Part model, mm, in its own coordinate system. A direction names the side the tool comes from. Round coordinates to 2 decimals unless told otherwise and drop trailing zeros. Loops run counter-clockwise (first coordinate to the right, second up) from the corner with the lowest first, then second, coordinate; pieces in that order, holes last. Notation, with made-up numbers: (-2, -32.5) - (30, -32.5) arc R7 cw to (30, -26.5) - close; hole circle Ø9 at (65.5, -38). An arc over 180 degrees is marked (long way). Put each result on its own line as item: value.
from build123d import *

# Parameters (mm, degrees)
EXTRUDE_1_DEPTH     = 65
MM_1_D              = 8
SKETCH_5_R          = 4.5
CUT_EXTRUDE_1_DEPTH = 89.741196746
SKETCH_6_R          = 7.5
CUT_EXTRUDE_2_DEPTH = 10
SKETCH_7_R          = 3.4
SKETCH_7_R_2        = 4
CUT_EXTRUDE_3_DEPTH = 24


with BuildPart() as part:
    # 草图1 → 凸台-拉伸1 (new body)
    with BuildSketch(Plane.XY):
        Polygon((-30, 44.5), (-30, 25), (0, 25), (0, 0), (-55, 0), (-55, 44.5), align=None)
    extrude(amount=EXTRUDE_1_DEPTH)

    # 大小mm 暗销孔1 (through all)
    with Locations(Plane(origin=(0, 25, 0), x_dir=(1, 0, 0), z_dir=(0, 1, 0))):
        with Locations((-12.5, -10), (-12.5, -40)):
            Hole(MM_1_D / 2)

    # 草图5 → 切除-拉伸1 (cut, through all)
    with BuildSketch(Plane(origin=(0, 25, 0), x_dir=(1, 0, 0), z_dir=(0, 1, 0))):
        with Locations(Location((-12.5, -25, 0), (0, 0, 270))):
            Circle(SKETCH_5_R)
        with Locations(Location((-12.5, -55, 0), (0, 0, 270))):
            Circle(SKETCH_5_R)
    extrude(amount=-CUT_EXTRUDE_1_DEPTH, mode=Mode.SUBTRACT)

    # 草图6 → 切除-拉伸2 (cut)
    with BuildSketch(Plane.XZ):
        with Locations((-12.5, 55)):
            Circle(SKETCH_6_R)
        with Locations((-12.5, 25)):
            Circle(SKETCH_6_R)
    extrude(amount=-CUT_EXTRUDE_2_DEPTH, mode=Mode.SUBTRACT)

    # 草图7 → 切除-拉伸3 (cut)
    with BuildSketch(Plane.ZY.offset(55)):
        with Locations((10, 32)):
            Circle(SKETCH_7_R)
        with Locations((25, 32)):
            Circle(SKETCH_7_R_2)
        with Locations((40, 32)):
            Circle(SKETCH_7_R)
        with Locations((55, 32)):
            Circle(SKETCH_7_R_2)
    extrude(amount=-CUT_EXTRUDE_3_DEPTH, mode=Mode.SUBTRACT)


solid = part.part
1. Band-saw the part on C-C (z = 25). List the corners of the cut face in (x, y).
A:
outline: (-55, 0) - (-20, 0) - (-20, 10) - (-17, 10) - (-17, 25) - (-30, 25) - (-30, 44.5) - (-55, 44.5) - (-55, 36) - (-31, 36) - (-31, 28) - (-55, 28) - close; (-8, 10) - (-5, 10) - (-5, 0) - (0, 0) - (0, 25) - (-8, 25) - close
2. Tool access for faces 4 (the flat face through (-33, 18, 0)), 5 (the flat face through (-43, 44.5, 32)), 6 (the flat face through (-7.6, 10, 25.1)), 7 (the cylindrical face through (-43.17, 30.7, 43.14)), 8 (the flat face through (-15, 25, 32)): list every direction of +Z, -Z, +X, -X, +Y, -Y with a clear straight run to the whole face (end or side of a thin tool).
A:
face 4: -Z, +X, -X, +Y, -Y
face 5: +Z, -Z, +X, -X, +Y
face 6: -Y
face 7: -X
face 8: +Z, -Z, +X, +Y
3. Pin check, flat tips, straight feed: P1, Ø12, axis at x = -12.5, z = 55, coming from the -Y side; P2, Ø4, axis at y = 33.5, z = 54, coming from the -X side; P3, Ø15.5, axis at y = 37.5, z = 47, coming from the +X side. Stop position of each tip, or through.
A:
P1: stops at y = 10
P2: stops at x = -31
P3: stops at x = -30
4. Two-plate mould, pull along X, no slides. Class faces 1 (the cylindrical face through (-13.476, 4.93, 32.436)), 2 (the flat face through (0, 13, 32)), 3 (the flat face through (-27, 0, 32)): pulls with the +X half, pulls with the -X half, needs draft (parallel to the pull), parting line crosses it, or undercut.
A:
face 1: undercut
face 2: pulls with the +X half
face 3: needs draft
5. Band-saw the part on D-D (x = -47.5). List the corners of the cut face in (y, z).
A:
outline: (0, 0) - (44.5, 0) - (44.5, 65) - (0, 65) - close; hole circle Ø8 at (32, 25); hole circle Ø8 at (32, 55); hole circle Ø6.8 at (32, 10); hole circle Ø6.8 at (32, 40)
6. Band-saw the part on B-B (y = 19). List the corners of the cut face in (x, z), plus the area to 3 significant figures.
A:
outline: (-55, 0) - (0, 0) - (0, 65) - (-55, 65) - close; hole circle Ø9 at (-12.5, 25); hole circle Ø9 at (-12.5, 55); hole circle Ø8 at (-12.5, 10); hole circle Ø8 at (-12.5, 40)
area: 3,350 mm²
7. Probe line 1 along X through (y, z) = (15, 40); line 2 along Y through (x, z) = (-39.5, 40); line 3 along Z through (x, y) = (-12, 8). List the from-to ranges inside material, lowest first. Write a range as [from, to].
A:
line 1: x = [-55, -16.5], [-8.5, 0]
line 2: y = [0, 28.6], [35.4, 44.5]
line 3: z = [0, 6.03], [13.97, 17.52], [32.48, 36.03], [43.97, 47.52], [62.48, 65]
8. Band-saw the part on A-A (x = -12.5). List the corners of the cut face in (y, z), plus the area to 3 significant figures.
A:
outline: (0, 0) - (25, 0) - (25, 6) - (0, 6) - close; (0, 14) - (25, 14) - (25, 20.5) - (10, 20.5) - (10, 17.5) - (0, 17.5) - close; (0, 32.5) - (10, 32.5) - (10, 29.5) - (25, 29.5) - (25, 36) - (0, 36) - close; (0, 44) - (25, 44) - (25, 50.5) - (10, 50.5) - (10, 47.5) - (0, 47.5) - close; (0, 62.5) - (10, 62.5) - (10, 59.5) - (25, 59.5) - (25, 65) - (0, 65) - close
area: 655 mm²
